Geometry: see drawing. Coordinates: mm, zero at the bounding-box minimum. Give positions to 0.01 mm unless a question says otherwise; leave off trailing zeros. Loops run counter-clockwise (first coordinate to the right, second up) from the corner with the lowest first, then second, coordinate; pieces in that order, holes last. Notation, with made-up numbers: (53, 8.25) - (63, 8.25) arc R30 cw to (63, 31.25) - close; hole circle Ø8 at (-38.5, -23). An arc over 180 degrees is marked (long way). Use one line per item in the form item = value.
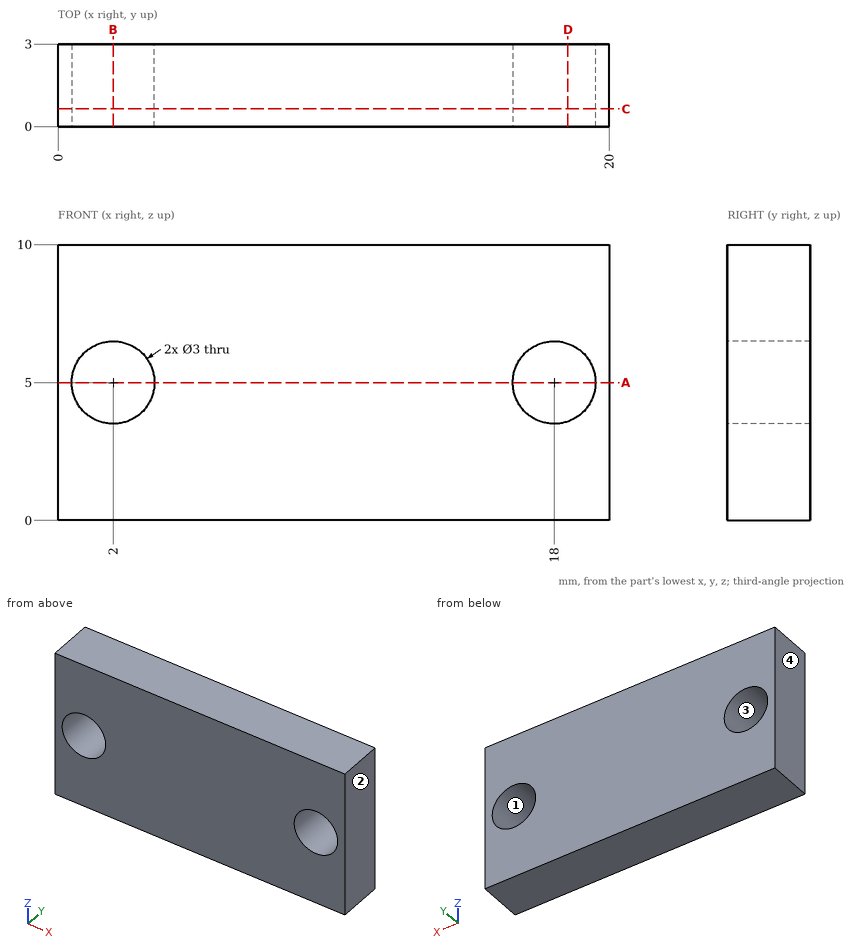
(1) Cut plane D-D (x = 18.5). Return the cut outline in (y, z).
Solution:
outline = (0, 0) - (3, 0) - (3, 3.59) - (0, 3.59) - close; (0, 6.41) - (3, 6.41) - (3, 10) - (0, 10) - close
(2) Cut plane B-B (x = 2). Return the cut outline in (y, z).
Solution:
outline = (0, 0) - (3, 0) - (3, 3.5) - (0, 3.5) - close; (0, 6.5) - (3, 6.5) - (3, 10) - (0, 10) - close
(3) Cut plane A-A (z = 5). Return the cut outline in (x, y), plus the area to 3 significant figures.
Solution:
outline = (0, 0) - (0.5, 0) - (0.5, 3) - (0, 3) - close; (3.5, 0) - (16.5, 0) - (16.5, 3) - (3.5, 3) - close; (19.5, 0) - (20, 0) - (20, 3) - (19.5, 3) - close
area = 42.0 mm2
(4) Cut plane C-C (y = 0.65). Return the cut outline in (x, z), plus the area to 3 significant figures.
Solution:
outline = (0, 0) - (20, 0) - (20, 10) - (0, 10) - close; hole circle Ø3 at (2, 5); hole circle Ø3 at (18, 5)
area = 186 mm2
(5) Pin query (flat end, axial travel): P1, Ø4, axis at x = 10, z = 6.5, coming from the -Y side. Return the tip coordinate at first contact, or that it passes through.
Solution:
P1 = 0
(6) Material intervals for L1, parallel to Z at x = 2, y = 1.95; L2, parallel to X at y = 2.15, z = 4.25; L3, parallel to X at y = 0.3, z = 4.75, sorted ascending. Write a range as from..to.
Solution:
L1 = 0..3.5, 6.5..10
L2 = 0..0.7, 3.3..16.7, 19.3..20
L3 = 0..0.52, 3.48..16.52, 19.48..20
(7) Pull-direction query (X, two-part tool) for the marked faces 1, 2, 3 and 4; classes: released by +X, released by -X, zero draft, split by the parting line, or undercut.
Solution:
face_1 = undercut
face_2 = released by +X
face_3 = undercut
face_4 = released by -X
